Input: dimensioned drawing with shaded views. Units: mm. Origin: part minimum x, y, z. A direction names the side the tool comes from. Give positions to 0.01 mm unless a question says otherwise; leave off trailing zeros. Write each loop counter-clockwise with the first axis right and the second up, starting at its lowest first coordinate (ties: lowest second). Pieces come first, ordered by that corner, then holes.
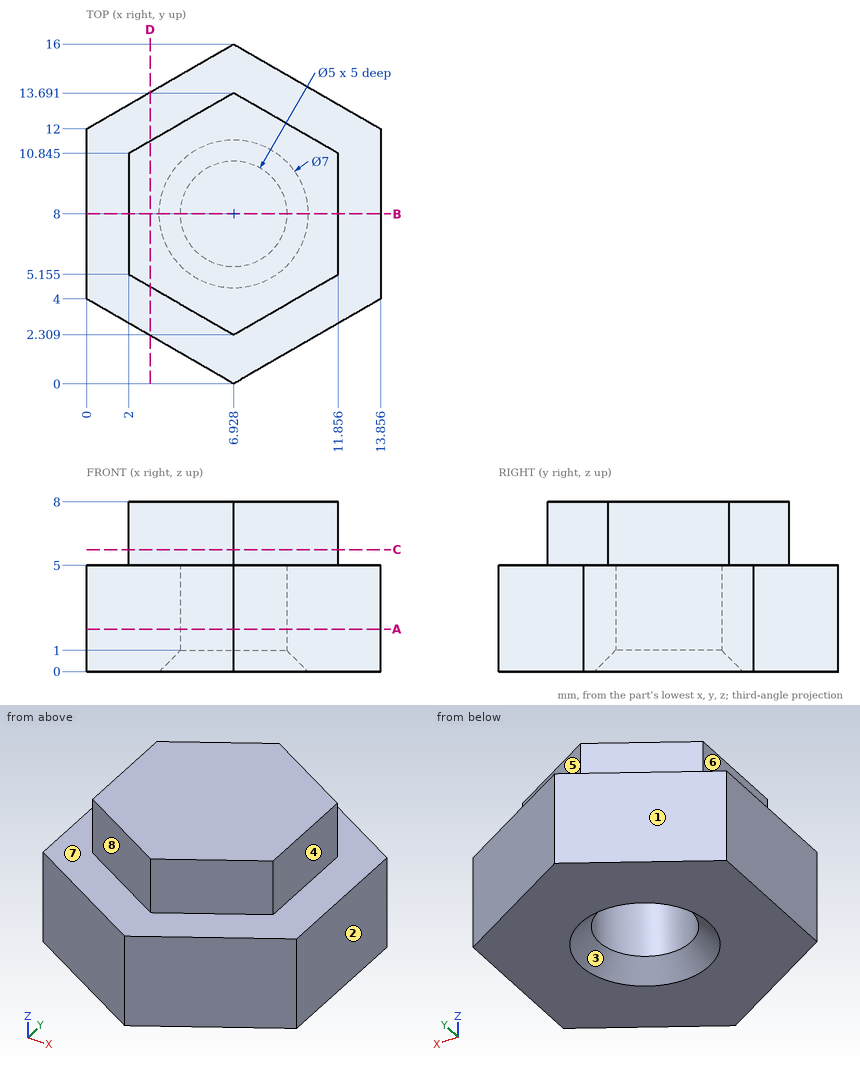
Item 1: Reachability of the marked faces 4, 5, 6, 7 and 8 from +Z, -Z, +X, -X, +Y, -Y: full face, straight path, thin tool, end or side. Return the list, or none.
Found:
face 4: +Z, +X, +Y, -Y
face 5: +Z, +X, +Y
face 6: +Z, -X, +Y, -Y
face 7: +Z
face 8: +Z, -X, -Y
Item 2: Section D-D, the plane x = 3. Return the cut outline in (y, z).
Found:
outline: (2.27, 0) - (13.73, 0) - (13.73, 5) - (11.42, 5) - (11.42, 8) - (4.58, 8) - (4.58, 5) - (2.27, 5) - close
Item 3: Line query: L1, parallel to Z at x = 7.75, y = 1.75; L2, parallel to X at y = 6.5, z = 6.75; L3, parallel to Z at x = 8, y = 6. Output: solid intervals per line, ascending.
Found:
L1: z = 0 to 5
L2: x = 2 to 11.86
L3: z = 5 to 8
Item 4: Section B-B, the plane y = 8. Return the cut outline in (x, z).
Found:
outline: (0, 0) - (3.43, 0) - (4.43, 1) - (4.43, 5) - (9.43, 5) - (9.43, 1) - (10.43, 0) - (13.86, 0) - (13.86, 5) - (11.86, 5) - (11.86, 8) - (2, 8) - (2, 5) - (0, 5) - close
Item 5: Pin query (flat end, axial travel): pin 1 Ø1.5 at (y, z) = (2.5, 1.5) entering from +X (1 decimal); pin 2 Ø0.9 at (y, z) = (8.5, 6.5) entering from +X; pin 3 Ø0.9 at (y, z) = (6.5, 6) entering from -X. Return the tip coordinate at first contact, or that it passes through.
Found:
pin 1: stops at x = 12.6
pin 2: stops at x = 11.86
pin 3: stops at x = 2
Item 6: Section A-A, the plane z = 2. Return the cut outline in (x, y), plus the area to 3 significant figures.
Found:
outline: (0, 4) - (6.93, 0) - (13.86, 4) - (13.86, 12) - (6.93, 16) - (0, 12) - close; hole circle Ø5 at (6.93, 8)
area: 147 mm2
Item 7: Pull-direction query (Y, two-part tool) for the marked faces 1, 2 and 3; classes: +Y half, -Y half, draft (parallel to the pull), parting line (faces both ways), or undercut.
Found:
face 1: +Y half
face 2: draft
face 3: undercut
Item 8: Section C-C, the plane z = 5.75. Return the cut outline in (x, y) (1 decimal).
Found:
outline: (2, 5.2) - (6.9, 2.3) - (11.9, 5.2) - (11.9, 10.8) - (6.9, 13.7) - (2, 10.8) - close
